For this review, take the finished solid that the model builds, in its own axes (mm). Round coordinates to 2 decimals unless told otherwise and drop trailing zeros. Order: outer loops, then holes, each group sorted by start corner. A loop starts at its lowest first (then second) coordinate and runs counter-clockwise, first axis right, second up.
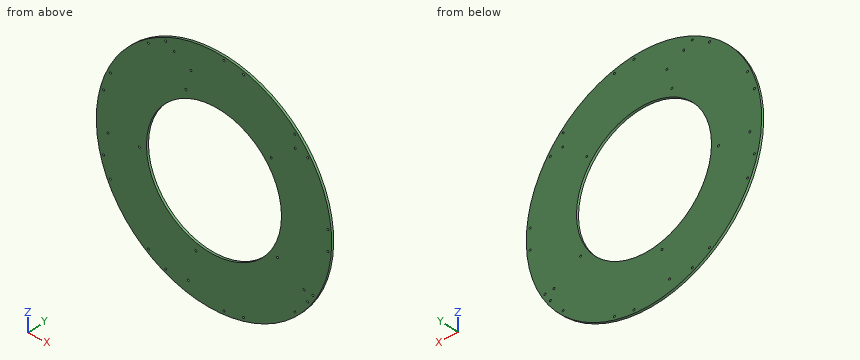
from build123d import *

# Parameters (mm, degrees)
SKETCH1_R                     = 309.88
SKETCH1_R_2                   = 177.8
BOSS_EXTRUDE1_DEPTH           = 5.842
SKETCH2_R                     = 2.5527
CUT_EXTRUDE1_DEPTH            = 439.275435958
CIRPATTERN1_COUNT             = 9
SKETCH3_R                     = 2.5527
HOLES_MOUNTINGFEET_DEPTH      = 439.275435958
CIRPATTERN_MOUNTINGFEET_COUNT = 5
SKETCH4_R                     = 2.5527
HOLE_WIRES_DEPTH              = 439.275435958
SKETCH5_R                     = 2.5527
CUT_EXTRUDE2_DEPTH            = 439.275435958


with BuildPart() as part:
    # Sketch1 → Boss-Extrude1 (new body)
    with BuildSketch(Plane(origin=(0, 0, 0), x_dir=(1, 0, 0), z_dir=(0, 1, 0))):
        with Locations(Location((0, 0, 0), (0, 0, 270))):
            Circle(SKETCH1_R)
        with Locations(Location((0, 0, 0), (0, 0, 270))):
            Circle(SKETCH1_R_2, mode=Mode.SUBTRACT)
    extrude(amount=BOSS_EXTRUDE1_DEPTH)

    # Sketch2 → Cut-Extrude1 (cut, through all)
    with BuildSketch(Plane(origin=(0, 5.842, 0), x_dir=(1, 0, 0), z_dir=(0, 1, 0))):
        with Locations(Location((-290.734014455, -77.901944385, 0), (0, 0, 270))):
            Circle(SKETCH2_R)
        with Locations(Location((-290.734014455, 77.901944385, 0), (0, 0, 270))):
            Circle(SKETCH2_R)
    cut_extrude1 = extrude(amount=-CUT_EXTRUDE1_DEPTH, mode=Mode.SUBTRACT)

    # CirPattern1: Cut-Extrude1 ×9 about axis
    cirpattern1_axis = Axis((0, 0, 0), (0, 1, 0))
    for i in range(1, CIRPATTERN1_COUNT):
        add(cut_extrude1.rotate(cirpattern1_axis, i * 360 / CIRPATTERN1_COUNT), mode=Mode.SUBTRACT)

    # Sketch3 → Holes_MountingFeet (cut, through all)
    with BuildSketch(Plane(origin=(0, 5.842, 0), x_dir=(1, 0, 0), z_dir=(0, 1, 0))):
        with Locations(Location((-196.370483294, 13.731561857, 0), (0, 0, 270))):
            Circle(SKETCH3_R)
        with Locations(Location((-278.719395643, 19.489958764, 0), (0, 0, 270))):
            Circle(SKETCH3_R)
    holes_mountingfeet = extrude(amount=-HOLES_MOUNTINGFEET_DEPTH, mode=Mode.SUBTRACT)

    # CirPattern_MountingFeet: Holes_MountingFeet ×5 about axis
    cirpattern_mountingfeet_axis = Axis((0, 0, 0), (0, 1, 0))
    for i in range(1, CIRPATTERN_MOUNTINGFEET_COUNT):
        add(holes_mountingfeet.rotate(cirpattern_mountingfeet_axis, i * 360 / CIRPATTERN_MOUNTINGFEET_COUNT), mode=Mode.SUBTRACT)

    # Sketch4 → Hole_Wires (cut, through all)
    with BuildSketch(Plane(origin=(0, 5.842, 0), x_dir=(1, 0, 0), z_dir=(0, 1, 0))):
        with Locations(Location((260.664986285, 150.495, 0), (0, 0, 270))):
            Circle(SKETCH4_R)
    extrude(amount=-HOLE_WIRES_DEPTH, mode=Mode.SUBTRACT)

    # Sketch5 → Cut-Extrude2 (cut, through all)
    with BuildSketch(Plane(origin=(0, 5.842, 0), x_dir=(1, 0, 0), z_dir=(0, 1, 0))):
        with Locations(Location((-60.478733235, -234.445699953, 0), (0, 0, 270))):
            Circle(SKETCH5_R)
    extrude(amount=-CUT_EXTRUDE2_DEPTH, mode=Mode.SUBTRACT)


solid = part.part
(1) Add section B-B on x = 0. Give the boundary of the cut face in (y, z).
(2) Add section A-A on z = 0. Give the boundary of the cut face in (x, y).
(3) Add section C-C on y = 1.9. Count the separate pieces of the cut face and the enclosed holes in it, plus the area to 3 significant figures.
(4) Clearance check with a flat-ended pin moving along its axis: P1, Ø1, axis at x = 217, y = 1.5, coming from the +Z side. State where the tip first meets the part, or that it passes through.
(5) Wall thickness on L1, parallel to X at y = 3.75, z = -14.5; L2, parallel to Z at x = -46.5, y = 5.05; L3, parallel to X at y = 2.9, z = 0: over which ranges is each line inside the solid? List them lowest first.
(6) Add section D-D on z = 224. Give the boundary of the cut face in (x, y), plus the area to 3 significant figures.
Here are the results:
1. outline: (0, -309.88) - (5.84, -309.88) - (5.84, -177.8) - (0, -177.8) - close; (0, 177.8) - (5.84, 177.8) - (5.84, 309.88) - (0, 309.88) - close
2. outline: (-309.88, 0) - (-177.8, 0) - (-177.8, 5.84) - (-309.88, 5.84) - close; (177.8, 0) - (309.88, 0) - (309.88, 5.84) - (177.8, 5.84) - close
3. separate pieces: 1
3. enclosed holes: 31
3. area: 202,000 mm2
4. P1: stops at z = 221.71
5. L1: x = -309.54 to -198.8, -193.94 to -177.21, 177.21 to 309.54
5. L2: z = -306.37 to -193.3, -188.71 to -171.61, 171.61 to 306.37
5. L3: x = -309.88 to -177.8, 177.8 to 309.88
6. outline: (-214.13, 0) - (214.13, 0) - (214.13, 5.84) - (-214.13, 5.84) - close
6. area: 2,500 mm2
